Part model, mm, in its own coordinate system. Face numbers are marked on the shaded views. A direction names the side the tool comes from. Coordinates: 2 decimals unless noted, no trailing zeros. Write each loop counter-clockwise with the first axis right and the second up, starting at its lowest first coordinate (ties: lowest second). Pieces come first, ordered by that corner, then holes. Notation, with made-up numbers: (37, 9) - (83, 9) arc R10 cw to (83, 20) - close; hole circle Ø5 at (-37.75, -33). An arc over 180 degrees is marked (long way). Use one line per item in the form item = value. Start each with the question number.
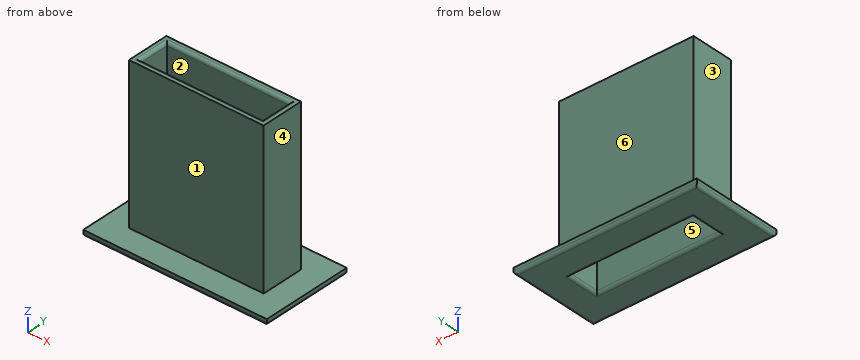
from build123d import *

# Parameters (mm, degrees)
F0_W     = 60
F0_H     = 30
F1_DEPTH = 2
F2_W     = 44
F2_H     = 14
F3_DEPTH = 50
F4_W     = 40
F4_H     = 10
F5_DEPTH = 52.001
F6_R     = 1


with BuildPart() as f1:
    # F0 (on Top) → F1 (new body)
    with BuildSketch(Plane.XY):
        Rectangle(F0_W, F0_H)
    extrude(amount=F1_DEPTH)

    # F2 (on face) → F3 (join)
    with BuildSketch(Plane.XY.offset(2)):
        Rectangle(F2_W, F2_H)
    extrude(amount=F3_DEPTH)

    # F4 (on face) → F5 (cut, through all)
    with BuildSketch(Plane.XY.offset(52)):
        Rectangle(F4_W, F4_H)
    extrude(amount=-F5_DEPTH, mode=Mode.SUBTRACT)

    # F6
    f6_edges = [f1.edges().sort_by_distance(p)[0] for p in [
        (30, 0, 0),
        (0, -15, 0),
        (0, 15, 0),
        (-30, 0, 0),
        (20, 0, 0),
        (0, 5, 0),
        (-20, 0, 0),
        (0, -5, 0),
        (0, 5, 52),
        (-20, 0, 52),
        (0, -5, 52),
        (20, 0, 52),
    ]]
    fillet(f6_edges, radius=F6_R)


solid = f1.part
Q1. Pin check, flat tips, straight feed: P1, Ø8, axis at y = -1, z = 33, coming from the +X side; P2, Ø8, axis at y = 2.5, z = 36, coming from the -X side; P3, Ø1.5, axis at x = 0, z = 41.5, coming from the +Y side. Stop position of each tip, or through.
Q2. Slice it at D-D (x = 25). List the corners of the cut face in (y, z).
Q3. Mould opens along X. For the marked faces 4, 5 and 6 say: released by +X, released by -X, zero draft, split by the parting line, or undercut.
Q4. Slice it at A-A (x = 1.5). List the corners of the cut face in (y, z).
Q5. Which spindle directions (+Z, -Z, +X, -X, +Y, -Y) get a long thin tool onto all of the face, cutting with end or side? Do the marked faces 1, 2 and 3. Say none if no direction does.
Q6. Slice it at B-B (y = -0.75). List the corners of the cut face in (x, z).
Q7. Slice it at C-C (z = 13). List the corners of the cut face in (x, y), plus the area to 3 significant figures.
Q8. Drill centre lines: probe 1 along Y at (x, z) = (17, 46.5); probe 2 along X at (y, z) = (-3.25, 4.5); probe 3 along Z at (x, y) = (1, 13.5). Where is each one in solid material? Low to high.
Solution:
q1.P1 = 22
q1.P2 = -22
q1.P3 = 7
q2.outline = (-15, 1) arc R1 ccw to (-14, 0) - (14, 0) arc R1 ccw to (15, 1) - (15, 2) - (-15, 2) - close
q3.face_4 = released by +X
q3.face_5 = undercut
q3.face_6 = zero draft
q4.outline = (-15, 1) arc R1 ccw to (-14, 0) - (-6, 0) arc R1 ccw to (-5, 1) - (-5, 51) arc R1 ccw to (-6, 52) - (-7, 52) - (-7, 2) - (-15, 2) - close; (5, 1) arc R1 ccw to (6, 0) - (14, 0) arc R1 ccw to (15, 1) - (15, 2) - (7, 2) - (7, 52) - (6, 52) arc R1 ccw to (5, 51) - close
q5.face_1 = +Z, +X, -X, -Y
q5.face_2 = +Z, -Z
q5.face_3 = +Z, -X, +Y, -Y
q6.outline = (-30, 1) arc R1 ccw to (-29, 0) - (-21, 0) arc R1 ccw to (-20, 1) - (-20, 51) arc R1 ccw to (-21, 52) - (-22, 52) - (-22, 2) - (-30, 2) - close; (20, 1) arc R1 ccw to (21, 0) - (29, 0) arc R1 ccw to (30, 1) - (30, 2) - (22, 2) - (22, 52) - (21, 52) arc R1 ccw to (20, 51) - close
q7.outline = (-22, -7) - (22, -7) - (22, 7) - (-22, 7) - close; hole (-20, -5) - (20, -5) - (20, 5) - (-20, 5) - close
q7.area = 216 mm2
q8.probe_1 = -7 to -5, 5 to 7
q8.probe_2 = -22 to -20, 20 to 22
q8.probe_3 = 0 to 2
